Source: CAD feature listing. Evaluate the final solid. Frame: model axes, mm. Face numbers are marked on the shaded views. Round coordinates to 2 decimals unless told otherwise and drop trailing zeros. Order: outer loops, then holes, each group sorted by start corner. A loop starts at its lowest first (then second) coordinate and runs counter-clockwise, first axis right, second up. Notation, with made-up numbers: (58, -20.5) -> (115, -20.5) arc R23 cw to (115, 11.5) -> close; hole circle Ø3 at (2, 4). An arc over 180 degrees is marked (long way). Answer as CSV lines item,"result".
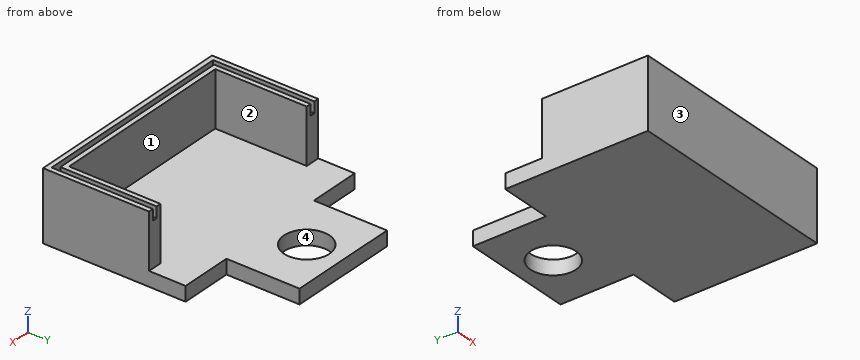
from build123d import *

# Parameters (mm, degrees)
SKETCH1_W           = 30.5
SKETCH1_H           = 20
SKETCH1_R           = 6.2
BOSS_EXTRUDE1_DEPTH = 4
SKETCH2_W           = 59
SKETCH2_H           = 4
BOSS_EXTRUDE2_DEPTH = 35
SKETCH4_W           = 59
SKETCH4_H           = 4
BOSS_EXTRUDE3_DEPTH = 4
SKETCH5_W           = 4
SKETCH5_H           = 25
BOSS_EXTRUDE4_DEPTH = 15
SKETCH6_W           = 1.333333334
SKETCH6_H           = 26.333333333
CUT_EXTRUDE1_DEPTH  = 3


with BuildPart() as part:
    # Sketch1 → Boss-Extrude1 (new body)
    with BuildSketch(Plane.XY):
        Rectangle(SKETCH1_W, SKETCH1_H)
        Circle(SKETCH1_R, mode=Mode.SUBTRACT)
    extrude(amount=BOSS_EXTRUDE1_DEPTH)

    # Sketch2 → Boss-Extrude2 (add)
    with BuildSketch(Plane.XZ.offset(10)):
        with Locations((0, 2)):
            Rectangle(SKETCH2_W, SKETCH2_H)
    extrude(amount=BOSS_EXTRUDE2_DEPTH)

    # Sketch4 → Boss-Extrude3 (add)
    with BuildSketch(Plane.XZ.offset(45)):
        with Locations((0, 2)):
            Rectangle(SKETCH4_W, SKETCH4_H)
    extrude(amount=BOSS_EXTRUDE3_DEPTH)

    # Sketch5 → Boss-Extrude4 (add)
    with BuildSketch(Plane.XY.offset(4)):
        with Locations((-27.5, -32.5)):
            Rectangle(SKETCH5_W, SKETCH5_H)
        Polygon((-29.5, -45), (-29.5, -49), (29.5, -49), (29.5, -45), (25.5, -45), (-25.5, -45), align=None)
        with Locations((27.5, -32.5)):
            Rectangle(SKETCH5_W, SKETCH5_H)
    extrude(amount=BOSS_EXTRUDE4_DEPTH)

    # Sketch6 → Cut-Extrude1 (cut)
    with BuildSketch(Plane.XY.offset(19)):
        Polygon((-26.833333333, -20), (-28.166666667, -20), (-28.166666667, -47.666666667), (-26.833333333, -47.666666667), (-26.833333333, -46.333333333), align=None)
        Polygon((26.833333333, -46.333333333), (-26.833333333, -46.333333333), (-26.833333333, -47.666666667), (28.166666667, -47.666666667), (28.166666667, -46.333333333), align=None)
        with Locations((27.5, -33.166666667)):
            Rectangle(SKETCH6_W, SKETCH6_H)
    extrude(amount=-CUT_EXTRUDE1_DEPTH, mode=Mode.SUBTRACT)


solid = part.part
1. Pin query (flat end, axial travel): pin 1 (4.5 mm diameter, centred on x = -23.5, z = 2.5, fed in from +Y); pin 2 (1.2 mm diameter, centred on y = -4, z = 1, fed in from -X); pin 3 (4.5 mm diameter, centred on x = 28.5, z = 8.5, fed in from +Y); pin 4 (3 mm diameter, centred on y = 2, z = 6, fed in from -X). Return the tip coordinate at first contact, or that it passes through.
Results below:
pin 1,"y = -10"
pin 2,"x = -15.25"
pin 3,"y = -20"
pin 4,"through"
2. Section query A-A on x = 0. Return loops of the section in (y, z).
Results below:
outline,"(-49, 0) -> (-6.2, 0) -> (-6.2, 4) -> (-45, 4) -> (-45, 19) -> (-46.33, 19) -> (-46.33, 16) -> (-47.67, 16) -> (-47.67, 19) -> (-49, 19) -> close; (6.2, 0) -> (10, 0) -> (10, 4) -> (6.2, 4) -> close"
3. Line query: L1, parallel to X at y = -23.5, z = 5.25; L2, parallel to Y at x = 0, z = 1.5; L3, parallel to Z at x = -27, y = -27. Output: solid intervals per line, ascending. Write a range as [from, to].
Results below:
L1,"[-29.5, -25.5], [25.5, 29.5]"
L2,"[-49, -6.2], [6.2, 10]"
L3,"[0, 16]"
4. Section query B-B on z = 17.5. Return loops of the section in (x, y), and give its area (3 significant figures).
Results below:
outline,"(-29.5, -49) -> (29.5, -49) -> (29.5, -20) -> (28.17, -20) -> (28.17, -47.67) -> (-28.17, -47.67) -> (-28.17, -20) -> (-29.5, -20) -> close; (-26.83, -46.33) -> (26.83, -46.33) -> (26.83, -20) -> (25.5, -20) -> (25.5, -45) -> (-25.5, -45) -> (-25.5, -20) -> (-26.83, -20) -> close"
area,"291 mm2"
5. Section query C-C on y = 0. Return loops of the section in (x, z).
Results below:
outline,"(-15.25, 0) -> (-6.2, 0) -> (-6.2, 4) -> (-15.25, 4) -> close; (6.2, 0) -> (15.25, 0) -> (15.25, 4) -> (6.2, 4) -> close"
6. Section query D-D on z = 1.75. Return loops of the section in (x, y), and give its area (3 significant figures).
Results below:
outline,"(-29.5, -49) -> (29.5, -49) -> (29.5, -10) -> (15.25, -10) -> (15.25, 10) -> (-15.25, 10) -> (-15.25, -10) -> (-29.5, -10) -> close; hole circle Ø12.4 at (0, 0)"
area,"2,790 mm2"
7. Mould query, pull axis Y, two halves, no side actions, for the marked faces 1, 2, 3 and 4. Classes: released by +Y, released by -Y, zero draft, split by the parting line, or undercut.
Results below:
face 1,"released by +Y"
face 2,"zero draft"
face 3,"released by -Y"
face 4,"undercut"
